Drawing for the job (mm, zero at the part's lowest x, y, z). A direction names the side the tool comes from. Coordinates: 2 decimals unless noted, no trailing zeros. Order: outer loops, then holes, each group sorted by start corner. A loop starts at its lowest first (then second) coordinate and runs counter-clockwise, first axis right, second up. Notation, with made-up numbers: M 31.25,65.25 L 78.25,65.25 A17 ccw 78.25,88.25 Z; hole C 79.25,88 d4. An arc over 180 degrees is marked long. Write item = value, one per line. Start each with the question number.
Q1. Band-saw the part on D-D on y = 6.75. Write the cut outline in (x, z).
Q2. Band-saw the part on A-A on y = 2.5. Write the cut outline in (x, z).
Q3. Band-saw the part on B-B on z = 1.25. Write the cut outline in (x, y).
Q4. Band-saw the part on C-C on x = 7.5. Write the cut outline in (y, z), plus the area to 3 significant figures.
Q5. Pull direction X, two halves, no side cores. Call the marked faces 4, 5, 6 and 7: released by +X, released by -X, zero draft, split by the parting line, or undercut.
Q6. Drill centre lines: probe 1 along X at (y, z) = (2, 4.25); probe 2 along Y at (x, z) = (5.25, 1.5); probe 3 along Y at (x, z) = (5.25, 4). Where is each one in solid material? Low to high.
Q7. Pin check, flat tips, straight feed: P1, Ø0.9, axis at x = 3.5, z = 3, coming from the -Y side; P2, Ø0.5, axis at x = 6.5, z = 0.5, coming from the +Y side; P3, Ø3.5, axis at x = 3.5, z = 2, coming from the +Y side. Stop position of each tip, or through.
Q8. 3-axis set-ups, long thin cutter, end or side, ignore diameter. For the marked faces 1, 2 and 3: which of +Z, -Z, +X, -X, +Y, -Y reach the whole face in a straight line?
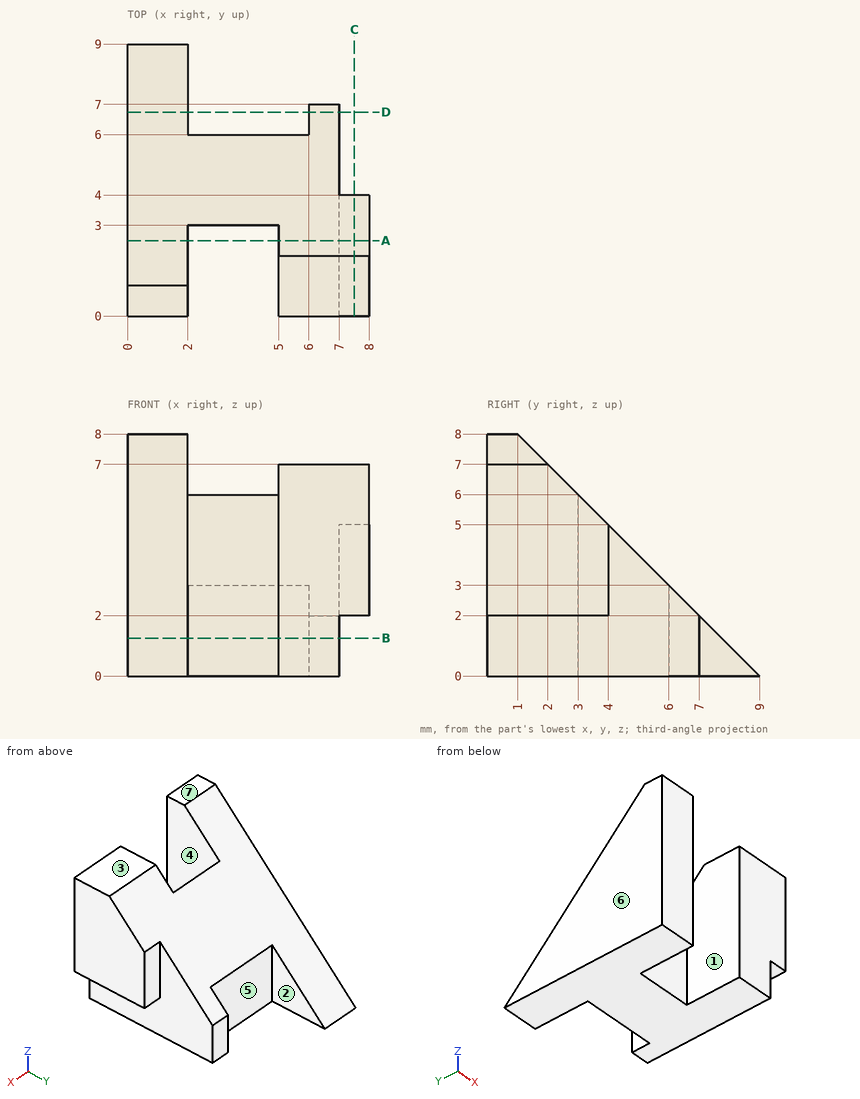
Recorded:
q1.outline = M 0,0 L 2,0 L 2,2.25 L 0,2.25 Z; M 6,0 L 7,0 L 7,2.25 L 6,2.25 Z
q2.outline = M 0,0 L 2,0 L 2,6.5 L 0,6.5 Z; M 5,0 L 7,0 L 7,2 L 8,2 L 8,6.5 L 5,6.5 Z
q3.outline = M 0,0 L 2,0 L 2,3 L 5,3 L 5,0 L 7,0 L 7,7 L 6,7 L 6,6 L 2,6 L 2,7.75 L 0,7.75 Z
q4.outline = M 0,2 L 4,2 L 4,5 L 2,7 L 0,7 Z
q4.area = 18.0 mm2
q5.face_4 = undercut
q5.face_5 = undercut
q5.face_6 = released by -X
q5.face_7 = zero draft
q6.probe_1 = 0 to 2, 5 to 8
q6.probe_2 = 0 to 6
q6.probe_3 = 0 to 5
q7.P1 = 3
q7.P2 = 7
q7.P3 = 7.9
q8.face_1 = +Z, -Z, -Y
q8.face_2 = +Z, -Z, +Y
q8.face_3 = +Z, +X, +Y, -Y
